```python
from build123d import *

# Parameters (mm, degrees)
SKETCH1_W           = 41
SKETCH1_H           = 41
SKETCH1_R           = 1.75
SKETCH1_R_2         = 1.25
BOSS_EXTRUDE1_DEPTH = 2
SKETCH2_W           = 10
SKETCH2_H           = 10
SKETCH2_R           = 1.75
BOSS_EXTRUDE2_DEPTH = 30
FILLET1_R           = 5
SKETCH3_R           = 10.5
CUT_EXTRUDE1_DEPTH  = 1
SKETCH4_R           = 11.5
CUT_EXTRUDE2_DEPTH  = 0.5


with BuildPart() as part:
    # Sketch1 → Boss-Extrude1 (new body)
    with BuildSketch(Plane.XY):
        with Locations((-34.508333333, 4.35625)):
            Rectangle(SKETCH1_W, SKETCH1_H)
        with Locations((-50.008333333, 19.85625)):
            Circle(SKETCH1_R, mode=Mode.SUBTRACT)
        with Locations((-50.008333333, -11.14375)):
            Circle(SKETCH1_R, mode=Mode.SUBTRACT)
        with Locations((-19.008333333, -11.14375)):
            Circle(SKETCH1_R, mode=Mode.SUBTRACT)
        with Locations((-19.008333333, 19.85625)):
            Circle(SKETCH1_R, mode=Mode.SUBTRACT)
        with Locations((-34.508333333, 4.35625)):
            Circle(SKETCH1_R_2, mode=Mode.SUBTRACT)
    extrude(amount=BOSS_EXTRUDE1_DEPTH)

    # Sketch2 → Boss-Extrude2 (add)
    # profile 1 of 4: a face of its own
    with BuildSketch(Plane.XY.offset(2)):
        with Locations((-50.008333333, 19.85625)):
            Rectangle(SKETCH2_W, SKETCH2_H)
        with Locations((-50.008333333, 19.85625)):
            Circle(SKETCH2_R, mode=Mode.SUBTRACT)
    # profile 2 of 4: a face of its own
    with BuildSketch(Plane.XY.offset(2)):
        with Locations((-50.008333333, -11.14375)):
            Rectangle(SKETCH2_W, SKETCH2_H)
        with Locations((-50.008333333, -11.14375)):
            Circle(SKETCH2_R, mode=Mode.SUBTRACT)
    # profile 3 of 4: a face of its own
    with BuildSketch(Plane.XY.offset(2)):
        with Locations((-19.008333333, -11.14375)):
            Rectangle(SKETCH2_W, SKETCH2_H)
        with Locations((-19.008333333, -11.14375)):
            Circle(SKETCH2_R, mode=Mode.SUBTRACT)
    # profile 4 of 4: a face of its own
    with BuildSketch(Plane.XY.offset(2)):
        with Locations((-19.008333333, 19.85625)):
            Rectangle(SKETCH2_W, SKETCH2_H)
        with Locations((-19.008333333, 19.85625)):
            Circle(SKETCH2_R, mode=Mode.SUBTRACT)
    extrude(amount=BOSS_EXTRUDE2_DEPTH)

    # Fillet1
    fillet1_edges = [part.edges().sort_by_distance(p)[0] for p in [
        (-24.008333333, 24.85625, 17),
        (-24.008333333, -6.14375, 17),
        (-55.008333333, -6.14375, 17),
        (-55.008333333, 14.85625, 17),
        (-45.008333333, 24.85625, 17),
        (-45.008333333, -6.14375, 17),
        (-45.008333333, -16.14375, 17),
        (-24.008333333, -16.14375, 17),
        (-14.008333333, -6.14375, 17),
        (-14.008333333, 14.85625, 17),
        (-24.008333333, 14.85625, 17),
        (-45.008333333, 14.85625, 17),
        (-14.008333333, -16.14375, 16),
        (-14.008333333, 24.85625, 16),
        (-55.008333333, -16.14375, 16),
        (-55.008333333, 24.85625, 16),
    ]]
    fillet(fillet1_edges, radius=FILLET1_R - 0.0001)  # a hair under: the kernel refuses the full size

    # Sketch3 → Cut-Extrude1 (cut)
    with BuildSketch(Plane.XY.offset(2)):
        with Locations((-34.508333333, 4.35625)):
            Circle(SKETCH3_R)
    extrude(amount=-CUT_EXTRUDE1_DEPTH, mode=Mode.SUBTRACT)

    # Sketch4 → Cut-Extrude2 (cut)
    with BuildSketch(Plane.XY.offset(2)):
        with Locations((-34.508333333, 4.35625)):
            Circle(SKETCH4_R)
    extrude(amount=-CUT_EXTRUDE2_DEPTH, mode=Mode.SUBTRACT)


solid = part.part
```
Can you work these out from the model? Positions are in its coordinate system, mm. A direction names the side the tool comes from. Coordinates: 2 decimals unless noted, no trailing zeros. Loops run counter-clockwise (first coordinate to the right, second up) from the corner with the lowest first, then second, coordinate; pieces in that order, holes last. Notation, with made-up numbers: (-28, -15.5) -> (-15, -15.5) arc R36 ccw to (-15, 18.5) -> close; hole circle Ø8 at (-38, 59.25). An arc over 180 degrees is marked (long way). Answer as a JSON object with one key per item and string values.
1) Imagine slicing it at A-A (y = -12). Please give me the cut outline in (x, z), then the cut area to 3 significant figures.
Results:
{"outline": "(-54.93, 0) -> (-51.53, 0) -> (-51.53, 32) -> (-54.93, 32) -> close; (-48.48, 0) -> (-20.53, 0) -> (-20.53, 32) -> (-23.93, 32) -> (-23.93, 2) -> (-45.08, 2) -> (-45.08, 32) -> (-48.48, 32) -> close; (-17.48, 0) -> (-14.08, 0) -> (-14.08, 32) -> (-17.48, 32) -> close", "area": "477 mm^2"}
2) Imagine slicing it at C-C (y = 21). Please give me the cut outline in (x, z).
Results:
{"outline": "(-54.88, 0) -> (-51.33, 0) -> (-51.33, 32) -> (-54.88, 32) -> close; (-48.68, 0) -> (-20.33, 0) -> (-20.33, 32) -> (-23.88, 32) -> (-23.88, 2) -> (-45.14, 2) -> (-45.14, 32) -> (-48.68, 32) -> close; (-17.68, 0) -> (-14.14, 0) -> (-14.14, 32) -> (-17.68, 32) -> close"}
3) Thinking about a two-plate mould opening in Y: for faces 4 (the face through (-46.43, 23.35, 17.21)), 5 (the face through (-55.008, 4, 1)), 6 (the face through (-29, -5, 1.5)), which applies, pulls with the +Y half, pulls with the -Y half, needs draft (parallel to the pull), parting line crosses it, or undercut?
Results:
{"face 4": "pulls with the +Y half", "face 5": "needs draft", "face 6": "undercut"}
4) If I drill on line 1 (Y direction, x = -50, z = 8); line 2 (X direction, y = 19, z = 26); line 3 (Z direction, x = -25, y = 1.5), over which ranges is the centre line in solid material (lowest first)?
Results:
{"line 1": "y = -16.14 to -12.89, -9.39 to -6.14, 14.86 to 18.11, 21.61 to 24.86", "line 2": "x = -54.93 to -51.53, -48.48 to -45.08, -23.93 to -20.53, -17.48 to -14.08", "line 3": "z = 0 to 1"}
5) For P1, Ø4, axis at y = -5, z = 24.5, coming from the +X side; P2, Ø12, axis at y = 20.5, z = 19, coming from the -X side; P3, Ø2, axis at x = -32.5, y = -11.5, coming from the +Z side; P4, Ø4, axis at x = -45.5, z = 10, coming from the +Y side, each with a flat end and sliding along its axis, tell me the tip position at first contact or that it passes through.
Results:
{"P1": "stops at x = -16.21", "P2": "stops at x = -55.01", "P3": "stops at z = 2", "P4": "stops at y = 24.18"}
6) For faces 1 (the face through (-35, 2, 1)), 2 (the face through (-15.434, 16.36, 17.21)), 3 (the face through (-53.583, -7.647, 17.21)), which set-ups out of +Z, -Z, +X, -X, +Y, -Y let a thin tool reach every point of the face, with its end or its side?
Results:
{"face 1": "+Z", "face 2": "+Z, +X", "face 3": "+Z, -X"}
7) Imagine slicing it at D-D (x = -41.5). Please give me the cut outline in (y, z).
Results:
{"outline": "(-16.14, 0) -> (24.86, 0) -> (24.86, 2) -> (13.49, 2) -> (13.49, 1.5) -> (12.19, 1.5) -> (12.19, 1) -> (-3.48, 1) -> (-3.48, 1.5) -> (-4.77, 1.5) -> (-4.77, 2) -> (-16.14, 2) -> close"}
8) Imagine slicing it at B-B (x = -34.5). Please give me the cut outline in (y, z).
Results:
{"outline": "(-16.14, 0) -> (3.11, 0) -> (3.11, 1) -> (-6.14, 1) -> (-6.14, 1.5) -> (-7.14, 1.5) -> (-7.14, 2) -> (-16.14, 2) -> close; (5.61, 0) -> (24.86, 0) -> (24.86, 2) -> (15.86, 2) -> (15.86, 1.5) -> (14.86, 1.5) -> (14.86, 1) -> (5.61, 1) -> close"}
